For this review, use the dimensioned drawing (mm, ordinates from the lowest corner) and the shaded views. A direction names the side the tool comes from. Round coordinates to 2 decimals unless told otherwise and drop trailing zeros. Write each loop counter-clockwise with the first axis right and the second up, starting at its lowest first coordinate (ties: lowest second). Pieces come first, ordered by that corner, then holes. Notation, with made-up numbers: M -16.75,38.25 L 32.25,38.25 A11 ccw 32.25,43.25 Z; hole C -26.75,-17 d1. An arc over 180 degrees is marked long. Write each question's results on one line, items separated by ' | '. Start each with the question number.
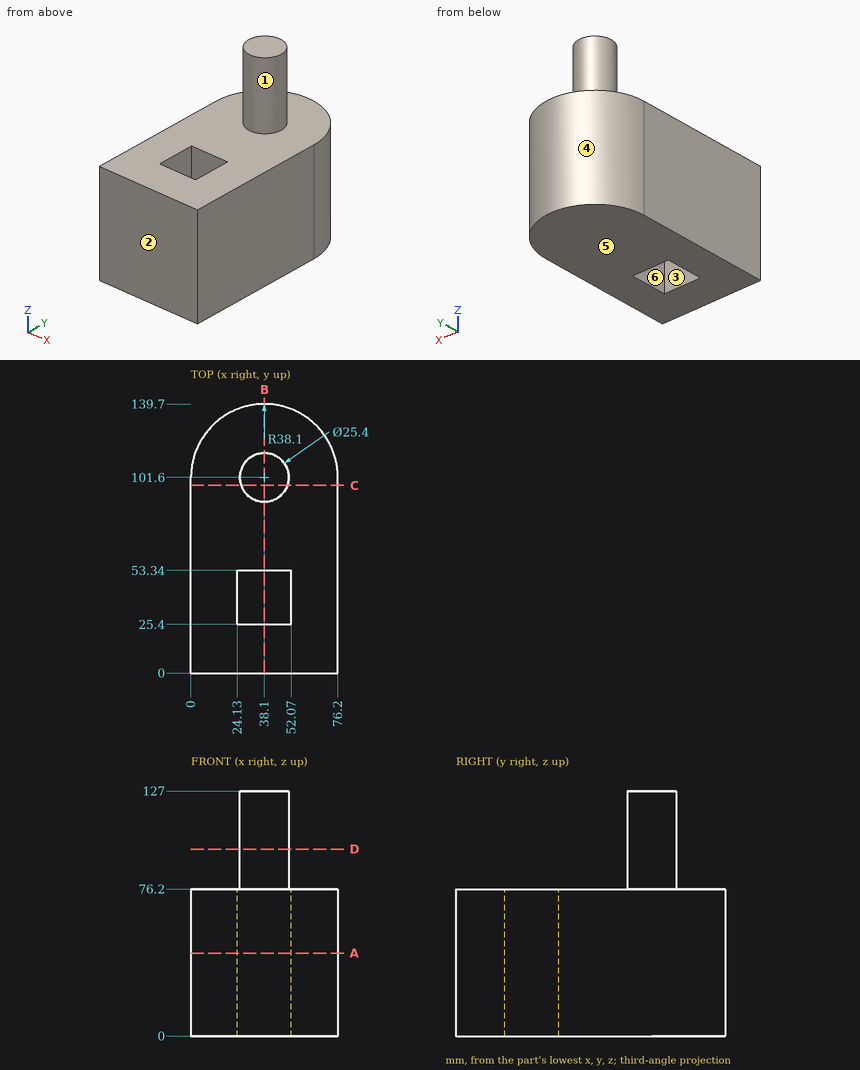
Item 1: Mouldability with a two-part tool opening along Y and no side actions: class the marked faces 4, 5 and 6 as pulls with the +Y half, pulls with the -Y half, needs draft (parallel to the pull), parting line crosses it, or undercut.
Item 2: For the marked faces 1, 2 and 3, list the 3-axis set-ups (+Z, -Z, +X, -X, +Y, -Y) from which the entire face can be reached by the end or side of a thin tool; tool diameter is ignored.
Item 3: We need section D-D on z = 97. State the section outline as (x, y) points, then the cut area to 3 significant figures.
Item 4: We need section B-B on x = 38.1. State the section outline as (y, z) points.
Item 5: We need section A-A on z = 43. State the section outline as (x, y) points.
Item 6: Insertion check: P1, Ø8.5, axis at x = 39.5, z = 35.5, coming from the +Y side; P2, Ø12, axis at x = 39, y = 79.5, coming from the +Z side; P3, Ø1.5, axis at y = 90, z = 100, coming from the +X side. Each pin has a flat end and moves straight along its axis. Give the tip position at first contact, or say it passes through.
Item 7: For probe 1 along X at (y, z) = (34.5, 5.5); probe 2 along Z at (x, y) = (29, 84.5); probe 3 along Y at (x, z) = (34.5, 44), list the stretches that pass through material, from the lowest coordinate up.
Item 8: We need section C-C on y = 97.5. State the section outline as (x, z) points, then the cut area to 3 significant figures.
Numbers:
1) face 4: pulls with the +Y half | face 5: needs draft | face 6: undercut
2) face 1: +Z | face 2: +Z, -Z, +X, -X, -Y | face 3: +Z, -Z
3) outline: C 38.1,101.6 d25.4 | area: 507 mm^2
4) outline: M 0,0 L 25.4,0 L 25.4,76.2 L 0,76.2 Z; M 53.34,0 L 139.7,0 L 139.7,76.2 L 114.3,76.2 L 114.3,127 L 88.9,127 L 88.9,76.2 L 53.34,76.2 Z
5) outline: M 0,0 L 76.2,0 L 76.2,101.6 A38.1 ccw 0,101.6 Z; hole M 24.13,25.4 L 52.07,25.4 L 52.07,53.34 L 24.13,53.34 Z
6) P1: stops at y = 139.7 | P2: stops at z = 76.2 | P3: stops at x = 44.7
7) probe 1: x = 0 to 24.13, 52.07 to 76.2 | probe 2: z = 0 to 76.2 | probe 3: y = 0 to 25.4, 53.34 to 139.53
8) outline: M 0,0 L 76.2,0 L 76.2,76.2 L 50.12,76.2 L 50.12,127 L 26.08,127 L 26.08,76.2 L 0,76.2 Z | area: 7,030 mm^2
